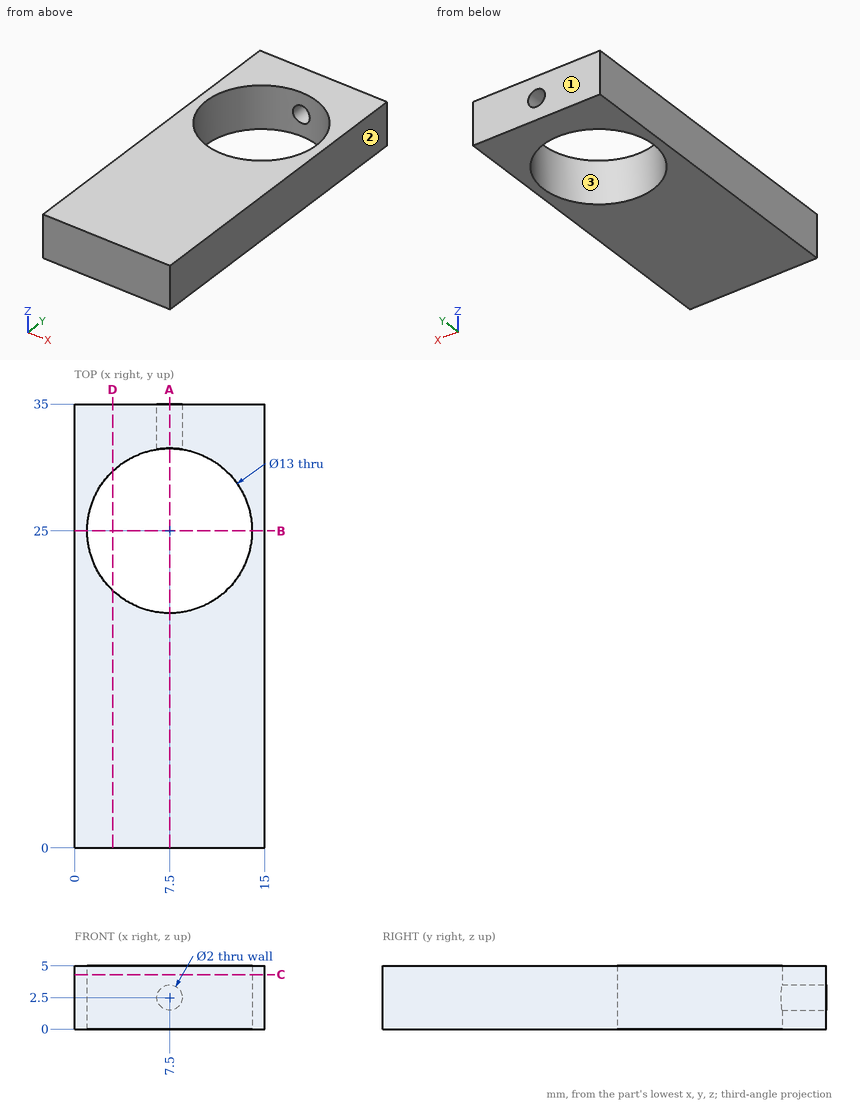
Answer from the drawing. Dimensions are ordinates in mm from the lowest x, y and z of the part. Round coordinates to 2 decimals unless told otherwise and drop trailing zeros. Loops run counter-clockwise (first coordinate to the right, second up) from the corner with the lowest first, then second, coordinate; pieces in that order, holes last.
Q1. This flat-tipped pin is pushed along its axis until it touches: pin 1 (3 mm diameter, centred on x = 13, z = 2, fed in from -Y). Where does it stop, or does it pass through?
Q2. Section D-D on x = 3 is taken. Write down the section's boundary in (y, z).
Q3. Consider probe 1 along Z at (x, y) = (7.5, 33.3); probe 2 along Y at (x, z) = (7.25, 0.25); probe 3 along Y at (x, z) = (10.25, 4.25). Determine where each line is inside the solid, lowest interval first.
Q4. Section C-C on z = 4.3 is taken. Write down the section's boundary in (x, y).
Q5. Section A-A on x = 7.5 is taken. Write down the section's boundary in (y, z), and give its area (3 significant figures).
Q6. Section B-B on y = 25 is taken. Write down the section's boundary in (x, z).
Q7. Determine the mould class of the marked faces 1, 2 and 3 for opening direction X: released by +X, released by -X, zero draft, split by the parting line, or undercut.
Output:
1. pin 1: stops at y = 0
2. outline: (0, 0) - (20.31, 0) - (20.31, 5) - (0, 5) - close; (29.69, 0) - (35, 0) - (35, 5) - (29.69, 5) - close
3. probe 1: z = 0 to 1.5, 3.5 to 5
3. probe 2: y = 0 to 18.5, 31.5 to 35
3. probe 3: y = 0 to 19.11, 30.89 to 35
4. outline: (0, 0) - (15, 0) - (15, 35) - (0, 35) - close; hole circle Ø13 at (7.5, 25)
5. outline: (0, 0) - (18.5, 0) - (18.5, 5) - (0, 5) - close; (31.5, 0) - (35, 0) - (35, 1.5) - (31.5, 1.5) - close; (31.5, 3.5) - (35, 3.5) - (35, 5) - (31.5, 5) - close
5. area: 103 mm2
6. outline: (0, 0) - (1, 0) - (1, 5) - (0, 5) - close; (14, 0) - (15, 0) - (15, 5) - (14, 5) - close
7. face 1: zero draft
7. face 2: released by +X
7. face 3: undercut
